Source: three-view drawing plus pictorial views. Frame: mm from the lowest corner of the part. A direction names the side the tool comes from. Coordinates: 2 decimals unless noted, no trailing zeros. Order: outer loops, then holes, each group sorted by start corner. A loop starts at its lowest first (then second) coordinate and runs counter-clockwise, first axis right, second up. Notation, with made-up numbers: (19.5, 35.25) - (67.5, 35.25) arc R22 cw to (67.5, 57.25) - close; hole circle Ø4 at (33.5, 73.25). An arc over 180 degrees is marked (long way). One line per question, with ' | ' between items.
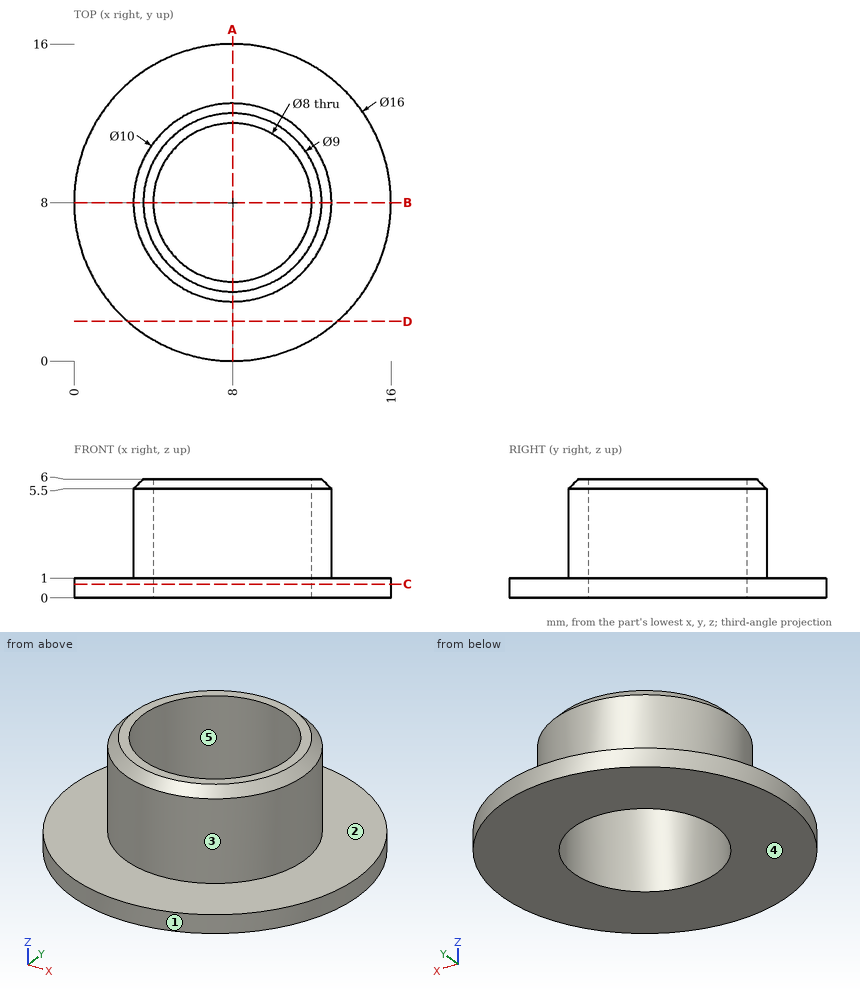
Item 1: Draft query along Y for the marked faces 3, 4 and 5. Return one class per face: released by +Y, released by -Y, zero draft, split by the parting line, or undercut.
Data:
face 3: split by the parting line | face 4: zero draft | face 5: undercut
Item 2: Section A-A on x = 8. Return the cut outline in (y, z).
Data:
outline: (0, 0) - (4, 0) - (4, 6) - (3.5, 6) - (3, 5.5) - (3, 1) - (0, 1) - close; (12, 0) - (16, 0) - (16, 1) - (13, 1) - (13, 5.5) - (12.5, 6) - (12, 6) - close
Item 3: Ray query, line 1 (Y direction, x = 8, z = 1.35); line 2 (Z direction, x = 10.5, y = 13.5); line 3 (X direction, y = 6.75, z = 3.2). Return the intervals inside material, ascending.
Data:
line 1: 3 to 4, 12 to 13 | line 2: 0 to 1 | line 3: 3.16 to 4.2, 11.8 to 12.84
Item 4: Contact query for flat-ended pins moving along their axis: P1, Ø1, axis at x = 4.5, z = 3, coming from the -Y side; P2, Ø3, axis at y = 13, z = 4.5, coming from the -X side; P3, Ø1.5, axis at x = 7.5, y = 5.5, coming from the +Z side. Output: stop coordinate, or through.
Data:
P1: y = 4 | P2: x = 4.43 | P3: through
Item 5: Access query for the marked faces 1 and 2. Directions: +Z, -Z, +X, -X, +Y, -Y. A direction counts if a zero-diameter tool reaches every point of the face in a straight line with its end or side. Return the directions, or none.
Data:
face 1: +Z, -Z | face 2: +Z
Item 6: Section C-C on z = 0.7. Return the cut outline in (x, y).
Data:
outline: circle Ø16 at (8, 8); hole circle Ø8 at (8, 8)
Item 7: Section D-D on y = 2. Return the cut outline in (x, z), and give its area (3 significant figures).
Data:
outline: (2.71, 0) - (13.29, 0) - (13.29, 1) - (2.71, 1) - close | area: 10.6 mm^2
